Here's how the part is built. I have some questions about the finished solid (model axes, mm). A direction names the side the tool comes from. Give positions to 0.01 mm unless a question says otherwise; leave off trailing zeros. Order: outer loops, then holes, each group sorted by start corner. A loop starts at its lowest first (then second) coordinate and runs counter-clockwise, first axis right, second up. Notation, with made-up numbers: (-6, -33) -> (31, -33) arc R17 cw to (31, -27) -> close; hole circle Ø7 at (15.25, -4). An arc over 180 degrees is marked (long way). Write each question's results on one line, items separated by ' | '. Start each with the question number.
Q1. I need wall thicknesses on line 1 along Y through (x, z) = (23, -15); line 2 along X through (y, z) = (6.25, 11); line 3 along Y through (x, z) = (24.5, 15.5). Which ranges of each line are inside material? Lowest first, please. Write a range as [from, to].
Q2. I'm going to push flat-ended pins straight in: pin 1 (1.6 mm diameter, centred on x = -0.5, y = 5.5, fed in from -Z); pin 2 (4 mm diameter, centred on x = 23, y = 5, fed in from -Z); pin 3 (1.6 mm diameter, centred on x = -0.5, y = 5.5, fed in from +Z). Where does each tip first touch, or does it pass through?
Q3. Imagine slicing it at A-A, the plane z = 10.5. Please give me the cut outline in (x, y).
Q4. Imagine slicing it at C-C, the plane y = 5. Please give me the cut outline in (x, z).
Q5. Imagine slicing it at D-D, the plane x = 22.5. Please give me the cut outline in (y, z).
Q6. Thinking about a two-plate mould opening in Y: for faces 1 (the face through (-0.4, 3.4, -12.6)), 2 (the face through (0, 10, 0)), 3 (the face through (0, 3, -17.5)), which applies, pulls with the +Y half, pulls with the -Y half, needs draft (parallel to the pull), parting line crosses it, or undercut?
Q7. For faces 4 (the face through (35, 5, 0)), 5 (the face through (-24.65, 5.07, 12.57)), 6 (the face through (0, 5, -7.5)), which set-ups out of +Z, -Z, +X, -X, +Y, -Y let a thin tool reach every point of the face, with its end or its side?
Q8. Imagine slicing it at B-B, the plane x = 0. Please give me the cut outline in (y, z), then the cut area to 3 significant figures.
```python
from build123d import *

# Parameters (mm, degrees)
SKETCH1_W           = 70
SKETCH1_H           = 35
BOSS_EXTRUDE1_DEPTH = 10
SKETCH2_R           = 1.65
CUT_EXTRUDE1_DEPTH  = 10


with BuildPart() as part:
    # Sketch1 → Boss-Extrude1 (new body)
    with BuildSketch(Plane(origin=(0, 0, 0), x_dir=(1, 0, 0), z_dir=(0, 1, 0))):
        Rectangle(SKETCH1_W, SKETCH1_H)
    extrude(amount=BOSS_EXTRUDE1_DEPTH)

    # Sketch2 → Cut-Extrude1 (cut)
    with BuildSketch(Plane.XY.offset(17.5)):
        with Locations((0, 5)):
            Circle(SKETCH2_R)
        with Locations((-23, 5)):
            Circle(SKETCH2_R)
        with Locations(Location((23, 5, 0), (0, 0, 180))):
            Circle(SKETCH2_R)
    cut_extrude1 = extrude(amount=-CUT_EXTRUDE1_DEPTH, mode=Mode.SUBTRACT)

    # Mirror1: Cut-Extrude1 across plane
    add(cut_extrude1.mirror(Plane.XY), mode=Mode.SUBTRACT)


solid = part.part
```
Geometry check:
1) line 1: [0, 3.35], [6.65, 10] | line 2: [-35, -24.08], [-21.92, -1.08], [1.08, 21.92], [24.08, 35] | line 3: [0, 4.31], [5.69, 10]
2) pin 1: z = -7.5 | pin 2: z = -17.5 | pin 3: z = 7.5
3) outline: (-35, 0) -> (35, 0) -> (35, 10) -> (-35, 10) -> close; hole circle Ø3.3 at (-23, 5); hole circle Ø3.3 at (0, 5); hole circle Ø3.3 at (23, 5)
4) outline: (-35, -17.5) -> (-24.65, -17.5) -> (-24.65, -7.5) -> (-21.35, -7.5) -> (-21.35, -17.5) -> (-1.65, -17.5) -> (-1.65, -7.5) -> (1.65, -7.5) -> (1.65, -17.5) -> (21.35, -17.5) -> (21.35, -7.5) -> (24.65, -7.5) -> (24.65, -17.5) -> (35, -17.5) -> (35, 17.5) -> (24.65, 17.5) -> (24.65, 7.5) -> (21.35, 7.5) -> (21.35, 17.5) -> (1.65, 17.5) -> (1.65, 7.5) -> (-1.65, 7.5) -> (-1.65, 17.5) -> (-21.35, 17.5) -> (-21.35, 7.5) -> (-24.65, 7.5) -> (-24.65, 17.5) -> (-35, 17.5) -> close
5) outline: (0, -17.5) -> (3.43, -17.5) -> (3.43, -7.5) -> (6.57, -7.5) -> (6.57, -17.5) -> (10, -17.5) -> (10, 17.5) -> (6.57, 17.5) -> (6.57, 7.5) -> (3.43, 7.5) -> (3.43, 17.5) -> (0, 17.5) -> close
6) face 1: undercut | face 2: pulls with the +Y half | face 3: needs draft
7) face 4: +Z, -Z, +X, +Y, -Y | face 5: +Z | face 6: -Z
8) outline: (0, -17.5) -> (3.35, -17.5) -> (3.35, -7.5) -> (6.65, -7.5) -> (6.65, -17.5) -> (10, -17.5) -> (10, 17.5) -> (6.65, 17.5) -> (6.65, 7.5) -> (3.35, 7.5) -> (3.35, 17.5) -> (0, 17.5) -> close | area: 284 mm²
